```python
from build123d import *

# Parameters (mm, degrees)
HEX_2_DEPTH = 2.2098


with BuildPart() as part:
    # BodySke → BaseBody (revolve)
    with BuildSketch(Plane.XY):
        with BuildLine():
            Line((44.6278, 0), (44.6278, 2.41935))
            Line((44.6278, 2.41935), (43.87215, 3.175))
            Line((43.87215, 3.175), (3.3528, 3.175))
            Line((3.3528, 3.175), (3.3528, 5.5499))
            Line((3.3528, 5.5499), (2.5654, 5.5499))
            ThreePointArc((2.5654, 5.5499), (1.073764503, 4.355582759), (0, 2.77495))
            Line((0, 2.77495), (0, 0))
            Line((0, 0), (44.6278, 0))
        make_face()
    revolve(axis=Axis((0, 0, 0), (1, 0, 0)))

    # Sketch2 → PreBroach (revolve, cut)
    with BuildSketch(Plane.XY):
        Polygon((0, 1.9812), (2.2098, 1.9812), (3.353646353, 0), (0, 0), align=None)
    revolve(axis=Axis((0, 0, 0), (1, 0, 0)), mode=Mode.SUBTRACT)

    # Sketch3 → Hex 2 (cut)
    with BuildSketch(Plane(origin=(0, 0, 0), x_dir=(0, 0, -1), z_dir=(1, 0, 0))):
        Polygon((-1.9812, -1.143846353), (-1.9812, 1.143846353), (0, 2.287692707), (1.9812, 1.143846353), (1.9812, -1.143846353), (0, -2.287692707), align=None)
    extrude(amount=HEX_2_DEPTH, mode=Mode.SUBTRACT)


solid = part.part
```
Input: part model. Units: mm. Frame: model coordinates. A direction names the side the tool comes from. Coordinates: 2 decimals unless noted, no trailing zeros. Loops run counter-clockwise (first coordinate to the right, second up) from the corner with the lowest first, then second, coordinate; pieces in that order, holes last. Notation, with made-up numbers: (67.5, 86.5) -> (121.5, 86.5) arc R29 ccw to (121.5, 118.5) -> close; hole circle Ø2 at (72.5, -17.75). An arc over 180 degrees is marked (long way). Use a Markdown table: item, result.
1) Cut plane A-A (x = 38). Return the cut outline in (y, z) (3 decimals).
Results found:
| item | result |
|---|---|
| outline | circle Ø6.35 at (0, 0) |
2) Pull-direction query (Y, two-part tool) for faces 1 (the cylindrical face through (2.954, 5.127, -2.126)), 2 (the flat face through (44.628, 0, 0)), 3 (the flat face through (1.09, -1.72, 0.98)); classes: released by +Y, released by -Y, zero draft, split by the parting line, or undercut.
Results found:
| item | result |
|---|---|
| face 1 | split by the parting line |
| face 2 | zero draft |
| face 3 | undercut |
3) Access query for faces 4 (the flat face through (1.09, 1.71, 1)), 5 (the cylindrical face through (23.33, -0.69, -3.1)), 6 (the flat face through (0, -2, -1)). Directions: +Z, -Z, +X, -X, +Y, -Y. A direction counts if a zero-diameter tool reaches every point of the face in a straight line with its end or side. Return the directions, or none.
Results found:
| item | result |
|---|---|
| face 4 | -X |
| face 5 | +X |
| face 6 | +Z, -Z, -X, +Y, -Y |
4) Cut plane B-B (y = -4.75). Return the cut outline in (x, z).
Results found:
| item | result |
|---|---|
| outline | (2.57, -2.87) -> (3.35, -2.87) -> (3.35, 2.87) -> (2.57, 2.87) arc R4.31 ccw to start |
5) Contact query for flat-ended pins moving along their axis: pin 1 (2 mm diameter, centred on y = -4, z = 0.5, fed in from +X); pin 2 (3 mm diameter, centred on x = 26.5, z = 0.5, fed in from +Y) (3 decimals); pin 3 (0.7 mm diameter, centred on x = 1.5, y = 0, fed in from +Z); pin 4 (1 mm diameter, centred on x = 26, y = 4, fed in from +Z). Output: stop coordinate, or through.
Results found:
| item | result |
|---|---|
| pin 1 | stops at x = 44.02 |
| pin 2 | stops at y = 3.175 |
| pin 3 | stops at z = 5.07 |
| pin 4 | passes through |
6) Cut plane C-C (z = -4). Return the cut outline in (x, y).
Results found:
| item | result |
|---|---|
| outline | (2.57, -3.85) -> (3.35, -3.85) -> (3.35, 3.85) -> (2.57, 3.85) arc R5.02 ccw to start |
7) Material intervals for line 1 along X through (y, z) = (-1.25, -1); line 2 along Z through (x, y) = (27.5, 0) (3 decimals); line 3 along X through (y, z) = (-2, 3.5), sorted ascending. Write a range as from..to.
Results found:
| item | result |
|---|---|
| line 1 | x = 2.43..44.63 |
| line 2 | z = -3.175..3.175 |
| line 3 | x = 0.79..3.35 |
